from build123d import *

# Parameters (mm, degrees)
SKETCH2_R           = 105
SKETCH2_R_2         = 21.59
SKETCH2_R_3         = 2
BOSS_EXTRUDE2_DEPTH = 3.175


with BuildPart() as part:
    # Sketch2 → Boss-Extrude2 (new body)
    with BuildSketch(Plane(origin=(0, 0, 0), x_dir=(1, 0, 0), z_dir=(0, 1, 0))):
        Circle(SKETCH2_R)
        with Locations((0, 80)):
            Circle(SKETCH2_R_2, mode=Mode.SUBTRACT)
        with Locations((72.770559628, 33.23320104)):
            Circle(SKETCH2_R_2, mode=Mode.SUBTRACT)
        with Locations((79.18571535, -11.385187062)):
            Circle(SKETCH2_R_2, mode=Mode.SUBTRACT)
        with Locations((60.459965948, -52.388858716)):
            Circle(SKETCH2_R_2, mode=Mode.SUBTRACT)
        with Locations((22.538604547, -76.759437889)):
            Circle(SKETCH2_R_2, mode=Mode.SUBTRACT)
        with Locations((-22.538604547, -76.759437889)):
            Circle(SKETCH2_R_2, mode=Mode.SUBTRACT)
        with Locations((-60.459965948, -52.388858716)):
            Circle(SKETCH2_R_2, mode=Mode.SUBTRACT)
        with Locations((-79.18571535, -11.385187062)):
            Circle(SKETCH2_R_2, mode=Mode.SUBTRACT)
        with Locations((-72.770559628, 33.23320104)):
            Circle(SKETCH2_R_2, mode=Mode.SUBTRACT)
        with Locations((-43.251265396, 67.300282626)):
            Circle(SKETCH2_R_2, mode=Mode.SUBTRACT)
        with Locations((0, 7.62)):
            Circle(SKETCH2_R_3, mode=Mode.SUBTRACT)
        with Locations((6.599113577, -3.81)):
            Circle(SKETCH2_R_3, mode=Mode.SUBTRACT)
        with Locations((-6.599113577, -3.81)):
            Circle(SKETCH2_R_3, mode=Mode.SUBTRACT)
    extrude(amount=BOSS_EXTRUDE2_DEPTH)


solid = part.part
Design review of the part built by this model. Coordinates are the model's own, in mm. Round coordinates to 2 decimals unless told otherwise and drop trailing zeros. Write each loop counter-clockwise with the first axis right and the second up, starting at its lowest first coordinate (ties: lowest second). Pieces come first, ordered by that corner, then holes. Notation, with made-up numbers: (61.5, 16.25) -> (90.5, 16.25) arc R26 ccw to (90.5, 50.25) -> close; hole circle Ø7 at (-27, -13.75). An arc over 180 degrees is marked (long way). One line per item, written item: value. Start each with the question number.
Q1. Add section D-D (z = 63.5). Give the boundary of the cut face in (x, y) (3 decimals), then the cut area to 3 significant figures.
Q2. To check wall thickness, follow probe 1 along Z at (x, y) = (19, 0.4); probe 2 along X at (y, z) = (1.35, -7.62); probe 3 along Z at (x, y) = (75, 2.25). State the ranges of each line that lie inside material, in increasing order.
Q3. Add section B-B (z = -25). Give the boundary of the cut face in (x, y) (3 decimals).
Q4. Insertion check: P1, Ø3, axis at x = 0, z = -7.62, coming from the +Y side. The pin has a flat end and moves straight along its axis. Give the tip position at first contact, or say it passes through.
Q5. Add section C-C (y = 1.9). State how many separate pieces and enclosed holes the cut face has, then the cut area to 3 significant figures.
Q6. Add section A-A (x = -76). Give the boundary of the cut face in (y, z) (3 decimals), then the cut area to 3 significant figures.
Q7. The part is to be moulded in two halves that separate along X. For faces 1 (the face through (-10.932, 1.565, 58.555)), 2 (the face through (-1, 0, -1)), 3 (the face through (100.15, 1.57, -31.54)), say which applies: pulls with the +X half, pulls with the -X half, needs draft (parallel to the pull), parting line crosses it, or undercut.
Response:
1. outline: (-83.623, 0) -> (-78.971, 0) -> (-78.971, 3.175) -> (-83.623, 3.175) -> close; (-41.949, 0) -> (-39.577, 0) -> (-39.577, 3.175) -> (-41.949, 3.175) -> close; (-5.5, 0) -> (5.5, 0) -> (5.5, 3.175) -> (-5.5, 3.175) -> close; (39.577, 0) -> (41.949, 0) -> (41.949, 3.175) -> (39.577, 3.175) -> close; (78.971, 0) -> (83.623, 0) -> (83.623, 3.175) -> (78.971, 3.175) -> close
1. area: 79.5 mm^2
2. probe 1: z = -103.27 to -90.25, -69.75 to 55.46, 98.06 to 103.27
2. probe 2: x = -104.72 to -89.43, -68.94 to -2, 2 to 68.94, 89.43 to 104.72
2. probe 3: z = -73.48 to -54.71, -11.76 to -9.8, 32.57 to 36.43, 68.35 to 73.48
3. outline: (-101.98, 0) -> (-92.729, 0) -> (-92.729, 3.175) -> (-101.98, 3.175) -> close; (-52.812, 0) -> (52.812, 0) -> (52.812, 3.175) -> (-52.812, 3.175) -> close; (92.729, 0) -> (101.98, 0) -> (101.98, 3.175) -> (92.729, 3.175) -> close
4. P1: passes through
5. separate pieces: 1
5. enclosed holes: 13
5. area: 20,000 mm^2
6. outline: (0, -72.45) -> (3.175, -72.45) -> (3.175, -54.58) -> (0, -54.58) -> close; (0, -11.886) -> (3.175, -11.886) -> (3.175, -9.968) -> (0, -9.968) -> close; (0, 32.739) -> (3.175, 32.739) -> (3.175, 37.401) -> (0, 37.401) -> close; (0, 67.377) -> (3.175, 67.377) -> (3.175, 72.45) -> (0, 72.45) -> close
6. area: 93.7 mm^2
7. face 1: undercut
7. face 2: needs draft
7. face 3: parting line crosses it
